from build123d import *

# Parameters (mm, degrees)
EXTRUDE_1_DEPTH     = 15
SKETCH_2_R          = 2.5
CUT_EXTRUDE_1_DEPTH = 371.312368143
SKETCH_2_3_R        = 2.5
CUT_EXTRUDE_2_DEPTH = 371.312368143


with BuildPart() as part:
    # ｽｹｯﾁ1 → ﾎﾞｽ - 押し出し1 (new body)
    with BuildSketch(Plane.XY):
        Polygon((-220, 297.5), (220, 297.5), (-45, -297.5), (-220, -297.5), align=None)
    extrude(amount=EXTRUDE_1_DEPTH)

    # ｽｹｯﾁ2 → ｶｯﾄ - 押し出し1 (cut, through all)
    with BuildSketch(Plane.XY.offset(15)):
        with Locations((-170, 285)):
            Circle(SKETCH_2_R)
        with Locations((-9.725, 285)):
            Circle(SKETCH_2_R)
        with Locations((150.55, 285)):
            Circle(SKETCH_2_R)
    cut_extrude_1 = extrude(amount=-CUT_EXTRUDE_1_DEPTH, mode=Mode.SUBTRACT)

    # ｽｹｯﾁ2<3> → ｶｯﾄ - 押し出し2 (cut, through all)
    with BuildSketch(Plane.XY.offset(15)):
        with Locations((-207.5, 247.5)):
            Circle(SKETCH_2_3_R)
        with Locations((-207.5, 123.75)):
            Circle(SKETCH_2_3_R)
        with Locations((-207.5, 0)):
            Circle(SKETCH_2_3_R)
        with Locations((-207.5, -123.75)):
            Circle(SKETCH_2_3_R)
        with Locations((-207.5, -247.5)):
            Circle(SKETCH_2_3_R)
    extrude(amount=-CUT_EXTRUDE_2_DEPTH, mode=Mode.SUBTRACT)

    # ﾐﾗｰ1: ｶｯﾄ - 押し出し1 across plane
    add(cut_extrude_1.mirror(Plane.ZX), mode=Mode.SUBTRACT)


solid = part.part
The listing builds one solid part. Answer for the finished solid, in the listing's coordinates (mm). Coordinates: 2 decimals unless noted, no trailing zeros. Order: outer loops, then holes, each group sorted by start corner. A loop starts at its lowest first (then second) coordinate and runs counter-clockwise, first axis right, second up. Notation, with made-up numbers: (-37.5, 26) -> (-32.5, 26) arc R13 cw to (-32.5, 51) -> close; hole circle Ø4 at (43, 47). An arc over 180 degrees is marked (long way). Answer in a Markdown table with one row per item. Add a question column.
Item 1: Find section A-A (z = 4.75). State how many separate pieces and enclosed holes the cut face has, then the cut area to 3 significant figures.
Item 2: Each of these flat-tipped pins is pushed along its axis until it touches: P1, Ø6.5, axis at x = -207.5, y = 247.5, coming from the -Z side; P2, Ø1, axis at x = -41, z = 9.5, coming from the -Y side; P3, Ø4.5, axis at x = -207.5, y = -123.75, coming from the -Z side; P4, Ø3, axis at y = -230.5, z = 8, coming from the +X side. Where does it stop, or does it pass through?
Item 3: Find section B-B (y = 34). Write down the section's boundary in (x, z), then the cut area to 3 significant figures.
Item 4: Find section C-C (x = 136). Write down the section's boundary in (y, z), then the cut area to 3 significant figures.
Item 5: Find the intervals of material crossed by L1, parallel to Y at x = -207.5, z = 3.5; L2, parallel to X at y = 285, z = 3.75 (3 decimals); L3, parallel to X at y = -247.5, z = 5.75, in increasing order. Write a range as from..to.
Result set:
| question | item | result |
|---|---|---|
| 1 | separate pieces | 1 |
| 1 | enclosed holes | 9 |
| 1 | area | 183,000 mm² |
| 2 | P1 | stops at z = 0 |
| 2 | P2 | stops at y = -289.64 |
| 2 | P3 | passes through |
| 2 | P4 | stops at x = -14.49 |
| 3 | outline | (-220, 0) -> (102.64, 0) -> (102.64, 15) -> (-220, 15) -> close |
| 3 | area | 4,840 mm² |
| 4 | outline | (108.9, 0) -> (297.5, 0) -> (297.5, 15) -> (108.9, 15) -> close |
| 4 | area | 2,830 mm² |
| 5 | L1 | y = -297.5..-250, -245..-126.25, -121.25..-2.5, 2.5..121.25, 126.25..245, 250..297.5 |
| 5 | L2 | x = -220..-172.5, -167.5..-12.225, -7.225..148.05, 153.05..214.433 |
| 5 | L3 | x = -220..-210, -205..-22.73 |
